Verification items for the finished model (mm, model axes). Give positions to 0.01 mm unless a question says otherwise; leave off trailing zeros. Write each loop counter-clockwise with the first axis right and the second up, starting at its lowest first coordinate (ties: lowest second). Pieces come first, ordered by that corner, then holes. Notation, with made-up numbers: (53.25, 80) -> (86.25, 80) arc R22 ccw to (86.25, 103) -> close; hole circle Ø6 at (1.5, -6.5). An arc over 180 degrees is marked (long way). Answer as CSV lines item,"result".
```python
from build123d import *

# Parameters (mm, degrees)
SKETCH1_R           = 1
BOSS_EXTRUDE1_DEPTH = 0.25
SKETCH2_R           = 1
CUT_EXTRUDE1_DEPTH  = 4.5
FILLET1_R           = 6


with BuildPart() as part:
    # Sketch1 → Boss-Extrude1 (new body)
    with BuildSketch(Plane(origin=(0, 0, 0), x_dir=(1, 0, 0), z_dir=(0, 1, 0))):
        Polygon((-21.4, 26.5), (-20.9, 26.5), (-20.9, -23.5), (-15, -26.5), (15, -26.5), (20.9, -23.5), (20.9, 26.5), (21.4, 26.5), (21.4, 29.5), (20.4, 30.5), (-20.4, 30.5), (-21.4, 29.5), align=None)
        with Locations((-19.944365081, 29.181392426)):
            Circle(SKETCH1_R, mode=Mode.SUBTRACT)
        with Locations((19.944365081, 29.181392426)):
            Circle(SKETCH1_R, mode=Mode.SUBTRACT)
    extrude(amount=BOSS_EXTRUDE1_DEPTH)

    # Sketch2 → Cut-Extrude1 (cut)
    with BuildSketch(Plane(origin=(0, 0.25, 0), x_dir=(1, 0, 0), z_dir=(0, 1, 0))):
        with Locations((-2.084530189, 19.934465076)):
            Circle(SKETCH2_R)
        with Locations((2.084530189, 19.934465076)):
            Circle(SKETCH2_R)
    extrude(amount=-CUT_EXTRUDE1_DEPTH, mode=Mode.SUBTRACT)

    # Fillet1
    fillet1_edges = [part.edges().sort_by_distance(p)[0] for p in [
        (20.9, 0.125, 23.5),
        (-20.9, 0.125, 23.5),
    ]]
    fillet(fillet1_edges, radius=FILLET1_R)


solid = part.part
```
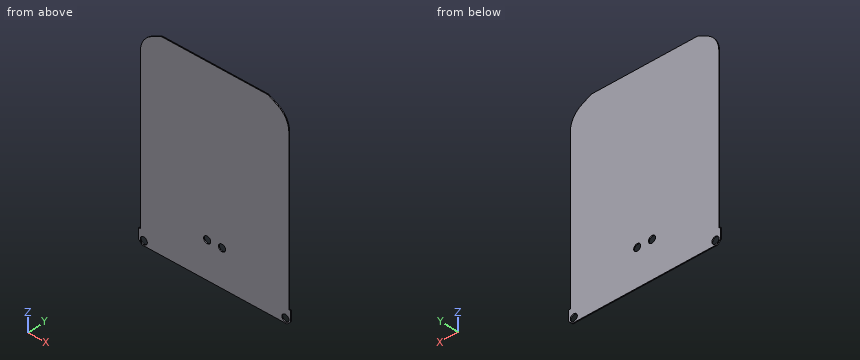
1) Section check A-A (y = 0.15). Record the boundary of the cut face in (x, z).
Reported:
outline,"(-21.4, -29.5) -> (-20.4, -30.5) -> (20.4, -30.5) -> (21.4, -29.5) -> (21.4, -26.5) -> (20.9, -26.5) -> (20.9, 19.82) arc R6 ccw to (17.62, 25.17) -> (15, 26.5) -> (-15, 26.5) -> (-17.62, 25.17) arc R6 ccw to (-20.9, 19.82) -> (-20.9, -26.5) -> (-21.4, -26.5) -> close; hole circle Ø2 at (-19.94, -29.18); hole circle Ø2 at (-2.08, -19.93); hole circle Ø2 at (2.08, -19.93); hole circle Ø2 at (19.94, -29.18)"
2) Section check B-B (z = -10). Record the boundary of the cut face in (x, y), and give its area (4 significant figures).
Reported:
outline,"(-20.9, 0) -> (20.9, 0) -> (20.9, 0.25) -> (-20.9, 0.25) -> close"
area,"10.45 mm²"
3) Depth check by flat-ended pin: pin 1 (1.6 mm diameter, centred on x = 19.94, z = -29.18, fed in from +Y). Enter the tip coordinate at first touch or a pass-through.
Reported:
pin 1,"through"
4) Scan lines: line 1 along X through (y, z) = (0.15, -1); line 2 along Z through (x, y) = (-17, 0.2); line 3 along Z through (x, y) = (-2.5, 0.05). Record each from-to range of solid material in increasing order.
Reported:
line 1,"-20.9 to 20.9"
line 2,"-30.5 to 25.48"
line 3,"-30.5 to -20.84, -19.02 to 26.5"
